```python
from build123d import *

# Parameters (mm, degrees)
BOSS_EXTRUDE1_DEPTH = 15
CUT_EXTRUDE1_REACH  = 17
SKETCH2_R           = 2.013136899


with BuildPart() as part:
    # Sketch1 → Boss-Extrude1 (new body)
    with BuildSketch(Plane(origin=(0, 0, 0), x_dir=(1, 0, 0), z_dir=(0, 1, 0))):
        with BuildLine():
            Line((-2.540599067, 15.797004665), (-1.5, 21))
            Line((-1.5, 21), (1.5, 21))
            Line((1.5, 21), (2.540599067, 15.797004665))
            ThreePointArc((2.540599067, 15.797004665), (4.141104722, 15.454813221), (5.698279, 14.950906877))
            Line((5.698279, 14.950906877), (9.200961894, 18.936533479))
            Line((9.200961894, 18.936533479), (11.799038106, 17.436533479))
            Line((11.799038106, 17.436533479), (10.098725665, 12.41030781))
            ThreePointArc((10.098725665, 12.41030781), (11.313708499, 11.313708499), (12.41030781, 10.098725665))
            Line((12.41030781, 10.098725665), (17.436533479, 11.799038106))
            Line((17.436533479, 11.799038106), (18.936533479, 9.200961894))
            Line((18.936533479, 9.200961894), (14.950906877, 5.698279))
            ThreePointArc((14.950906877, 5.698279), (15.454813221, 4.141104722), (15.797004665, 2.540599067))
            Line((15.797004665, 2.540599067), (21, 1.5))
            Line((21, 1.5), (21, -1.5))
            Line((21, -1.5), (15.797004665, -2.540599067))
            ThreePointArc((15.797004665, -2.540599067), (15.454813221, -4.141104722), (14.950906877, -5.698279))
            Line((14.950906877, -5.698279), (18.936533479, -9.200961894))
            Line((18.936533479, -9.200961894), (17.436533479, -11.799038106))
            Line((17.436533479, -11.799038106), (12.41030781, -10.098725665))
            ThreePointArc((12.41030781, -10.098725665), (11.313708499, -11.313708499), (10.098725665, -12.41030781))
            Line((10.098725665, -12.41030781), (11.799038106, -17.436533479))
            Line((11.799038106, -17.436533479), (9.200961894, -18.936533479))
            Line((9.200961894, -18.936533479), (5.698279, -14.950906877))
            ThreePointArc((5.698279, -14.950906877), (4.141104722, -15.454813221), (2.540599067, -15.797004665))
            Line((2.540599067, -15.797004665), (1.5, -21))
            Line((1.5, -21), (-1.5, -21))
            Line((-1.5, -21), (-2.540599067, -15.797004665))
            ThreePointArc((-2.540599067, -15.797004665), (-4.141104722, -15.454813221), (-5.698279, -14.950906877))
            Line((-5.698279, -14.950906877), (-9.200961894, -18.936533479))
            Line((-9.200961894, -18.936533479), (-11.799038106, -17.436533479))
            Line((-11.799038106, -17.436533479), (-10.098725665, -12.41030781))
            ThreePointArc((-10.098725665, -12.41030781), (-11.313708499, -11.313708499), (-12.41030781, -10.098725665))
            Line((-12.41030781, -10.098725665), (-17.436533479, -11.799038106))
            Line((-17.436533479, -11.799038106), (-18.936533479, -9.200961894))
            Line((-18.936533479, -9.200961894), (-14.950906877, -5.698279))
            ThreePointArc((-14.950906877, -5.698279), (-15.454813221, -4.141104722), (-15.797004665, -2.540599067))
            Line((-15.797004665, -2.540599067), (-21, -1.5))
            Line((-21, -1.5), (-21, 1.5))
            Line((-21, 1.5), (-15.797004665, 2.540599067))
            ThreePointArc((-15.797004665, 2.540599067), (-15.454813221, 4.141104722), (-14.950906877, 5.698279))
            Line((-14.950906877, 5.698279), (-18.936533479, 9.200961894))
            Line((-18.936533479, 9.200961894), (-17.436533479, 11.799038106))
            Line((-17.436533479, 11.799038106), (-12.41030781, 10.098725665))
            ThreePointArc((-12.41030781, 10.098725665), (-11.313708499, 11.313708499), (-10.098725665, 12.41030781))
            Line((-10.098725665, 12.41030781), (-11.799038106, 17.436533479))
            Line((-11.799038106, 17.436533479), (-9.200961894, 18.936533479))
            Line((-9.200961894, 18.936533479), (-5.698279, 14.950906877))
            ThreePointArc((-5.698279, 14.950906877), (-4.141104722, 15.454813221), (-2.540599067, 15.797004665))
        make_face()
    extrude(amount=BOSS_EXTRUDE1_DEPTH)

    # Sketch2 → Cut-Extrude1 (cut, up to next)
    with BuildSketch(Plane(origin=(0, 0, 0), x_dir=(1, 0, 0), z_dir=(0, 1, 0)), mode=Mode.PRIVATE) as cut_extrude1_sk1:
        Circle(SKETCH2_R)
    cut_extrude1_tool1 = extrude(cut_extrude1_sk1.sketch, amount=CUT_EXTRUDE1_REACH, mode=Mode.PRIVATE) & part.part
    add(cut_extrude1_tool1.solids().sort_by_distance((0, 0, 0))[0], mode=Mode.SUBTRACT)


solid = part.part
```
For this review, take the finished solid that the model builds, in its own axes (mm). A direction names the side the tool comes from. Coordinates: 2 decimals unless noted, no trailing zeros. Write each loop counter-clockwise with the first axis right and the second up, starting at its lowest first coordinate (ties: lowest second). Pieces come first, ordered by that corner, then holes.
(1) For pin 1 Ø1.5 at (x, y) = (8.5, 5.5) entering from +Z; pin 2 Ø4 at (y, z) = (8.5, -5.5) entering from +X; pin 3 Ø5 at (x, y) = (16, 8) entering from -Z, all flat-tipped, find the tip position at first contact; note any pin that passes through.
(2) The part is to be moulded in two halves that separate along X. For faces 1 (the face through (7.5, 7.4, 17)), 2 (the face through (21, 7, 0)), 3 (the face through (-16.92, 7.4, -7.43)), 4 (the face through (-14.96, 7.4, -10.96)), say which applies: +X half, -X half, draft (parallel to the pull), parting line (faces both ways), or undercut.
(3) Add section D-D on x = 6.5. Give the boundary of the cut face in (y, z).
(4) Add section A-A on z = 0. Give the boundary of the cut face in (x, y), then the cut area to 3 significant figures.
(5) Add section B-B on x = 0. Give the boundary of the cut face in (y, z).
(6) Wall thickness on probe 1 along Z at (x, y) = (0, 9.5); probe 2 along Z at (x, y) = (18, 4.75): over which ranges is each line inside the solid? List them lowest first.
(7) Add section C-C on x = -18. Give the boundary of the cut face in (y, z).
(8) Tool access review of faces 5 (the face through (-4, 15, 0)), 6 (the face through (11.33, 7.4, 11.3)), 7 (the face through (-7.5, 7.4, -17)), 8 (the face through (15.45, 7.4, -4.16)), 9 (the face through (-18.435, 7.395, -2.013)): name each direction out of +Z, -Z, +X, -X, +Y, -Y from which nothing blocks a thin tool from reaching the whole face with its end or side.
Answer sheet:
1. pin 1: stops at z = 18.94
1. pin 2: stops at x = 17
1. pin 3: stops at z = -11.8
2. face 1: undercut
2. face 2: +X half
2. face 3: -X half
2. face 4: undercut
3. outline: (0, -15.86) - (15, -15.86) - (15, 15.86) - (0, 15.86) - close
4. outline: (-21, 0) - (-2.01, 0) - (-2.01, 15) - (-21, 15) - close; (2.01, 0) - (21, 0) - (21, 15) - (2.01, 15) - close
4. area: 570 mm2
5. outline: (0, -21) - (15, -21) - (15, -2.01) - (0, -2.01) - close; (0, 2.01) - (15, 2.01) - (15, 21) - (0, 21) - close
6. probe 1: z = -21 to -2.01, 2.01 to 21
6. probe 2: z = -10.82 to -8.38, -2.1 to 2.1, 8.38 to 10.82
7. outline: (0, -10.82) - (15, -10.82) - (15, -8.38) - (0, -8.38) - close; (0, -2.1) - (15, -2.1) - (15, 2.1) - (0, 2.1) - close; (0, 8.38) - (15, 8.38) - (15, 10.82) - (0, 10.82) - close
8. face 5: +Z, -Z, +X, -X, +Y
8. face 6: +Y, -Y
8. face 7: -Z, +Y, -Y
8. face 8: +X, +Y, -Y
8. face 9: -X, +Y, -Y
